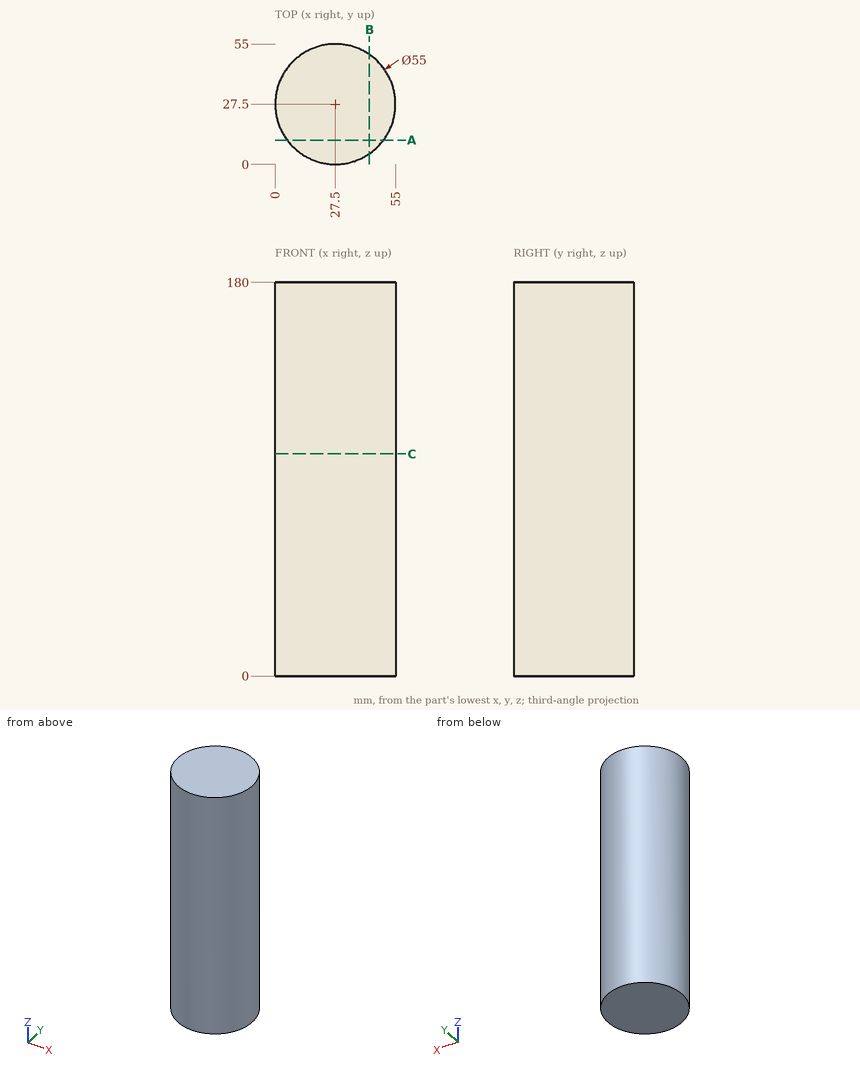
Design review of the part shown in the three views and the two pictorial views. Dimensions are in mm from the part's minimum x, y and z. Round coordinates to 2 decimals unless told otherwise and drop trailing zeros. Write each loop counter-clockwise with the first axis right and the second up, starting at its lowest first coordinate (ties: lowest second). Pieces come first, ordered by that corner, then holes. Notation, with made-up numbers: (50, 26) -> (97, 26) arc R27 ccw to (97, 63) -> close; hole circle Ø11 at (-7.75, 72.5). An arc over 180 degrees is marked (long way). Use one line per item in the form item = value.
1) Take a section at A-A, the plane y = 11. Write out the cut boundary in (x, z).
Found:
outline = (5.5, 0) -> (49.5, 0) -> (49.5, 180) -> (5.5, 180) -> close
2) Take a section at B-B, the plane x = 43. Write out the cut boundary in (y, z), and give its area (3 significant figures).
Found:
outline = (4.78, 0) -> (50.22, 0) -> (50.22, 180) -> (4.78, 180) -> close
area = 8,180 mm2
3) Clearance check with flat-ended pins moving along their axes: pin 1 (5 mm diameter, centred on x = 46.5, z = 31, fed in from +Y); pin 2 (8 mm diameter, centred on x = 22.5, z = 88.5, fed in from +Y); pin 3 (4 mm diameter, centred on y = 21, z = 32, fed in from +X). State where each tip first meets the part, or that it passes through.
Found:
pin_1 = 49.5
pin_2 = 54.98
pin_3 = 54.63
4) To check wall thickness, follow L1, parallel to X at y = 28.5, z = 113.5; L2, parallel to X at y = 34, z = 22.5. State the ranges of each line that lie inside material, in increasing order. Write a range as from..to.
Found:
L1 = 0.02..54.98
L2 = 0.78..54.22
5) Take a section at C-C, the plane z = 101.5. Write out the cut boundary in (x, y), and give its area (3 significant figures).
Found:
outline = circle Ø55 at (27.5, 27.5)
area = 2,380 mm2
